Can you work these out from the model? Positions are in its coordinate system, mm. A direction names the side the tool comes from. Round coordinates to 2 decimals unless told otherwise and drop trailing zeros. Loops run counter-clockwise (first coordinate to the right, second up) from the corner with the lowest first, then second, coordinate; pieces in that order, holes last. Notation, with made-up numbers: M 49.25,33.25 L 83.25,33.25 A24 cw 83.25,47.25 Z; hole C -12.75,-15 d1. An arc over 180 degrees is marked long. Answer as CSV lines item,"result".
from build123d import *
from OCP.BRepAlgoAPI import BRepAlgoAPI_Cut
from OCP.TopTools import TopTools_ListOfShape

# Parameters (mm, degrees)
SKETCH1_W               = 22.054431489
SKETCH1_H               = 12.5
BOSS_EXTRUDE1_DEPTH     = 43
CUT_EXTRUDE1_DEPTH      = 10
CUT_EXTRUDE1_DEPTH_BACK = 15
SKETCH2_R               = 1.5
FILLET3_START           = -1
FILLET3_DEPTH           = 42
FILLET3_START_2         = -31
FILLET3_2_DEPTH         = 14
SKETCH5_R               = 1.5
CUT_EXTRUDE4_DEPTH      = 57.301199739
SKETCH16_W              = 22.05443149
SKETCH16_H              = 2
CUT_EXTRUDE6_DEPTH      = 8.5
FILLET4_START           = -31
FILLET4_DEPTH           = 14


with BuildPart() as part:
    # Sketch1 → Boss-Extrude1 (new body)
    with BuildSketch(Plane.XY):
        with Locations((-13.228930986, -24.070183414)):
            Rectangle(SKETCH1_W, SKETCH1_H)
    extrude(amount=BOSS_EXTRUDE1_DEPTH)

    # Sketch2 → Cut-Extrude1 (cut, two sides: drawn at the far end of the back side and taken through both)
    with BuildSketch(Plane.XZ.offset(30.320183414).offset(-CUT_EXTRUDE1_DEPTH_BACK)):
        with Locations(Location((-13.228930986, 6.5, 0), (0, 0, 90))):
            Circle(SKETCH2_R)
        with Locations(Location((-13.228930986, 36.5, 0), (0, 0, 90))):
            Circle(SKETCH2_R)
        with BuildLine():
            Line((-3.524026068, 36.5), (-2.201715242, 36.5))
            add(Edge.make_bspline(
                [(-24.256146731, 33.845079723), (-30.410867424, 43.557524996), (-12.605557553, 54.855746483), (11.277296074, 42.57460591), (-2.201715242, 36.5)],
                knots=[0, 0, 0, 0, 0.503104745, 1, 1, 1, 1], degree=3))
            add(Edge.make_bspline(
                [(-3.83164653, 38.924092472), (-9.250736817, 38.125111697), (-28.532285754, 46.163812106), (-24.256146731, 33.845079723)],
                knots=[0, 0, 0, 0, 1, 1, 1, 1], degree=3))
            ThreePointArc((-3.83164653, 38.924092472), (-3.601238334, 37.721766617), (-3.524026068, 36.5))
        make_face()
        with BuildLine():
            Line((-4.478930986, 8.75), (-2.201715242, 8.75))
            add(Edge.make_bspline(
                [(-2.201715242, 8.75), (5.39210746, 3.880294823), (-0.777052631, -4.523329032), (-17.174300591, -10.623347238), (-34.821400648, -0.026005424), (-24.256146731, 8.75)],
                knots=[0, 0, 0, 0, 0.283272691, 0.504244858, 1, 1, 1, 1], degree=3))
            add(Edge.make_bspline(
                [(-23.490579314, 0), (-24.966512963, 4.237786421), (-24.256146731, 8.75)],
                knots=[0, 0, 0, 1, 1, 1], degree=2))
            Line((-23.490579314, 0), (-13.228930986, 0))
            ThreePointArc((-13.228930986, 0), (-7.041746651, 2.562815665), (-4.478930986, 8.75))
        make_face()
    extrude(amount=CUT_EXTRUDE1_DEPTH + CUT_EXTRUDE1_DEPTH_BACK, mode=Mode.SUBTRACT)


with BuildPart() as fillet3_tool:
    # Fillet3: read off the stored shape, not the designer's step
    # Fillet3 outline → Fillet3 (new body)
    with BuildSketch(Plane.XY.offset(FILLET3_START)):
        with BuildLine():
            Line((-24.256146731, -17.820183414), (-24.256146731, -19.820183414))
            ThreePointArc((-24.256146731, -19.820183414), (-23.670360293, -18.405969851), (-22.256146731, -17.820183414))
            Line((-22.256146731, -17.820183414), (-24.256146731, -17.820183414))
        make_face()
        with BuildLine():
            ThreePointArc((-22.256146731, -30.320183414), (-23.670360293, -29.734396976), (-24.256146731, -28.320183414))
            Line((-24.256146731, -28.320183414), (-24.256146731, -30.320183414))
            Line((-24.256146731, -30.320183414), (-22.256146731, -30.320183414))
        make_face()
    extrude(amount=FILLET3_DEPTH)


with BuildPart() as part_1:
    add(part.part)

    # Fillet3: cut by fillet3_tool, with a tolerance
    fillet3_stock = TopTools_ListOfShape()
    fillet3_stock.Append(part_1.part.wrapped)
    fillet3_tools = TopTools_ListOfShape()
    fillet3_tools.Append(fillet3_tool.part.wrapped)
    fillet3_cut = BRepAlgoAPI_Cut()
    fillet3_cut.SetArguments(fillet3_stock)
    fillet3_cut.SetTools(fillet3_tools)
    fillet3_cut.SetFuzzyValue(0.00001)
    fillet3_cut.Build()
    add(Compound.cast(fillet3_cut.Shape()).solids(), mode=Mode.REPLACE)


with BuildPart() as fillet3_2_tool:
    # Fillet3 2 outline → Fillet3 2 (new body)
    with BuildSketch(Plane(origin=(0, 0, 0), x_dir=(1, 0, 0), z_dir=(0, 1, 0)).offset(FILLET3_START_2)):
        with BuildLine():
            Line((-24.256146731, -3.001504812), (-24.256146731, -3.16929397))
            ThreePointArc((-24.256146731, -3.16929397), (-24.248700679, -2.996873655), (-24.226417966, -2.82573719))
            add(Edge.make_bspline(
                [(-24.226417966, -2.82573719), (-24.241732441, -2.913564505), (-24.256146731, -3.001504812)],
                knots=[0.329874436, 0.329874436, 0.329874436, 0.350165787, 0.350165787, 0.350165787], degree=2))
        make_face()
        with BuildLine():
            ThreePointArc((-23.275055203, -39.963216674), (-23.99364737, -39.232721814), (-24.256146731, -38.242221169))
            Line((-24.256146731, -38.242221169), (-24.256146731, -39.081457115))
            add(Edge.make_bspline(
                [(-24.256146731, -39.081457115), (-23.999461699, -39.439477902), (-23.668462552, -39.730301433), (-23.275055203, -39.963216674)],
                knots=[0.20342968, 0.20342968, 0.20342968, 0.20342968, 0.271697972, 0.271697972, 0.271697972, 0.271697972], degree=3))
        make_face()
    extrude(amount=FILLET3_2_DEPTH)


with BuildPart() as part_2:
    add(part_1.part)

    # Fillet3 2: cut by fillet3_2_tool, with a tolerance
    fillet3_2_stock = TopTools_ListOfShape()
    fillet3_2_stock.Append(part_2.part.wrapped)
    fillet3_2_tools = TopTools_ListOfShape()
    fillet3_2_tools.Append(fillet3_2_tool.part.wrapped)
    fillet3_2_cut = BRepAlgoAPI_Cut()
    fillet3_2_cut.SetArguments(fillet3_2_stock)
    fillet3_2_cut.SetTools(fillet3_2_tools)
    fillet3_2_cut.SetFuzzyValue(0.00001)
    fillet3_2_cut.Build()
    add(Compound.cast(fillet3_2_cut.Shape()).solids(), mode=Mode.REPLACE)

    # Sketch5 → Cut-Extrude4 (cut, through all)
    with BuildSketch(Plane.XY):
        with Locations(Location((-18.011106811, -24.070183414, 0), (0, 0, 180))):
            Circle(SKETCH5_R)
        with Locations(Location((-8.446755162, -24.070183414, 0), (0, 0, 180))):
            Circle(SKETCH5_R)
    extrude(amount=CUT_EXTRUDE4_DEPTH, mode=Mode.SUBTRACT)

    # Sketch16 → Cut-Extrude6 (cut)
    with BuildSketch(Plane.XY.offset(38)):
        with Locations((-13.228930985, -20.1809771)):
            Rectangle(SKETCH16_W, SKETCH16_H)
        with Locations((-13.228930985, -28.261916897)):
            Rectangle(SKETCH16_W, SKETCH16_H)
    extrude(amount=-CUT_EXTRUDE6_DEPTH, mode=Mode.SUBTRACT)

    # Fillet4: read off the stored shape, not the designer's step
    # Fillet4 outline → Fillet4 (cut)
    with BuildSketch(Plane(origin=(0, 0, 0), x_dir=(1, 0, 0), z_dir=(0, 1, 0)).offset(FILLET4_START)):
        with BuildLine():
            ThreePointArc((-3.536641618, -36.994677952), (-4.113301238, -38.300390358), (-5.413622589, -38.88910556))
            add(Edge.make_bspline(
                [(-5.413622589, -38.88910556), (-4.807642485, -38.852553426), (-4.273553237, -38.858938555), (-3.83164653, -38.924092472)],
                knots=[0.91845371, 0.91845371, 0.91845371, 0.91845371, 1, 1, 1, 1], degree=3))
            ThreePointArc((-3.83164653, -38.924092472), (-3.635515677, -37.966820429), (-3.536641618, -36.994677952))
        make_face()
    extrude(amount=FILLET4_DEPTH, mode=Mode.SUBTRACT)


solid = part_2.part
Item 1: If we section it at B-B on y = -20.25: State how many separate pieces and enclosed holes the cut face has, then the cut area to 3 significant figures.
Output:
separate pieces,"2"
enclosed holes,"1"
area,"645 mm2"
Item 2: On a 3-axis mill with a long thin cutter (end or side, diameter ignored), from which of +Z, -Z, +X, -X, +Y, -Y can I reach the whole of each face in a straight line? I mean faces 1 (the face through (-13, -21.181, 34)), 2 (the face through (-3, -24, 8.75)), 3 (the face through (-3, -18, 36.5)). Say none if no direction works.
Output:
face 1,"+X, -X"
face 2,"-Z, +X, +Y, -Y"
face 3,"+Z, +X, +Y, -Y"
Item 3: We'd pull the mould along X, two halves only. Please class faces 4 (the face through (-24.256, -24, 20)), 5 (the face through (-14.24, -24.18, 35.39)), 6 (the face through (-13, -19.181, 34)): released by +X, released by -X, zero draft, split by the parting line, or undercut.
Output:
face 4,"released by -X"
face 5,"undercut"
face 6,"zero draft"
Item 4: Will these pins go through, and if not, where does the flat tip stop? pin 1 (3.5 mm diameter, centred on x = -8.45, y = -24.07, fed in from +Z); pin 2 (6 mm diameter, centred on x = -14, y = -29, fed in from +Z); pin 3 (0.5 mm diameter, centred on x = -3, y = -30, fed in from +Z); pin 4 (0.6 mm diameter, centred on x = -15.5, y = -28, fed in from -Z).
Output:
pin 1,"stops at z = 39.58"
pin 2,"stops at z = 40.65"
pin 3,"stops at z = 36.5"
pin 4,"stops at z = 0"
Item 5: If we section it at C-C on z = 6.5: Write out the boundary of the cut face in (x, y).
Output:
outline,"M -24.26,-28.32 A2 ccw -22.26,-30.32 L -14.73,-30.32 L -14.73,-17.82 L -22.26,-17.82 A2 ccw -24.26,-19.82 Z; M -11.73,-30.32 L -4.77,-30.32 L -4.77,-17.82 L -11.73,-17.82 Z; hole C -18.01,-24.07 d3; hole C -8.45,-24.07 d3"
Item 6: If we section it at D-D on x = -5: Write out the boundary of the cut face in (y, z).
Output:
outline,"M -30.32,5.78 L -17.82,5.78 L -17.82,38.82 L -30.32,38.82 Z; hole M -29.26,29.5 L -27.26,29.5 L -27.26,38 L -29.26,38 Z; hole M -21.18,29.5 L -19.18,29.5 L -19.18,38 L -21.18,38 Z"
Item 7: If I drill on line 1 along Y through (x, z) = (-20.5, 37.5); line 2 along X through (y, z) = (-23.5, 33); line 3 along Z through (x, y) = (-13.25, -26.5), over which ranges is the centre line in solid material (lowest first)? Write a range as from..to.
Output:
line 1,"y = -30.32..-29.26, -27.26..-21.18, -19.18..-17.82"
line 2,"x = -24.26..-19.4, -16.62..-9.83, -7.06..-2.2"
line 3,"z = 0..5, 8..35, 38..40.12"
Item 8: If we section it at A-A on z = 30.5: Write out the boundary of the cut face in (x, y).
Output:
outline,"M -24.26,-27.26 L -2.2,-27.26 L -2.2,-21.18 L -24.26,-21.18 Z; M -24.15,-19.18 L -2.2,-19.18 L -2.2,-17.82 L -22.26,-17.82 A2 ccw Z; M -24.02,-29.26 A2 ccw -22.26,-30.32 L -2.2,-30.32 L -2.2,-29.26 Z; hole C -18.01,-24.07 d3; hole C -8.45,-24.07 d3"
